For this review, use the dimensioned drawing (mm, ordinates from the lowest corner) and the shaded views. A direction names the side the tool comes from. Coordinates: 2 decimals unless noted, no trailing zeros. Write each loop counter-clockwise with the first axis right and the second up, starting at its lowest first coordinate (ties: lowest second). Pieces come first, ordered by that corner, then holes. Notation, with made-up numbers: (71.5, 28) - (97.5, 28) arc R12 ccw to (97.5, 38) - close; hole circle Ø7 at (7, 50). An arc over 180 degrees is marked (long way). One line per item, written item: value.
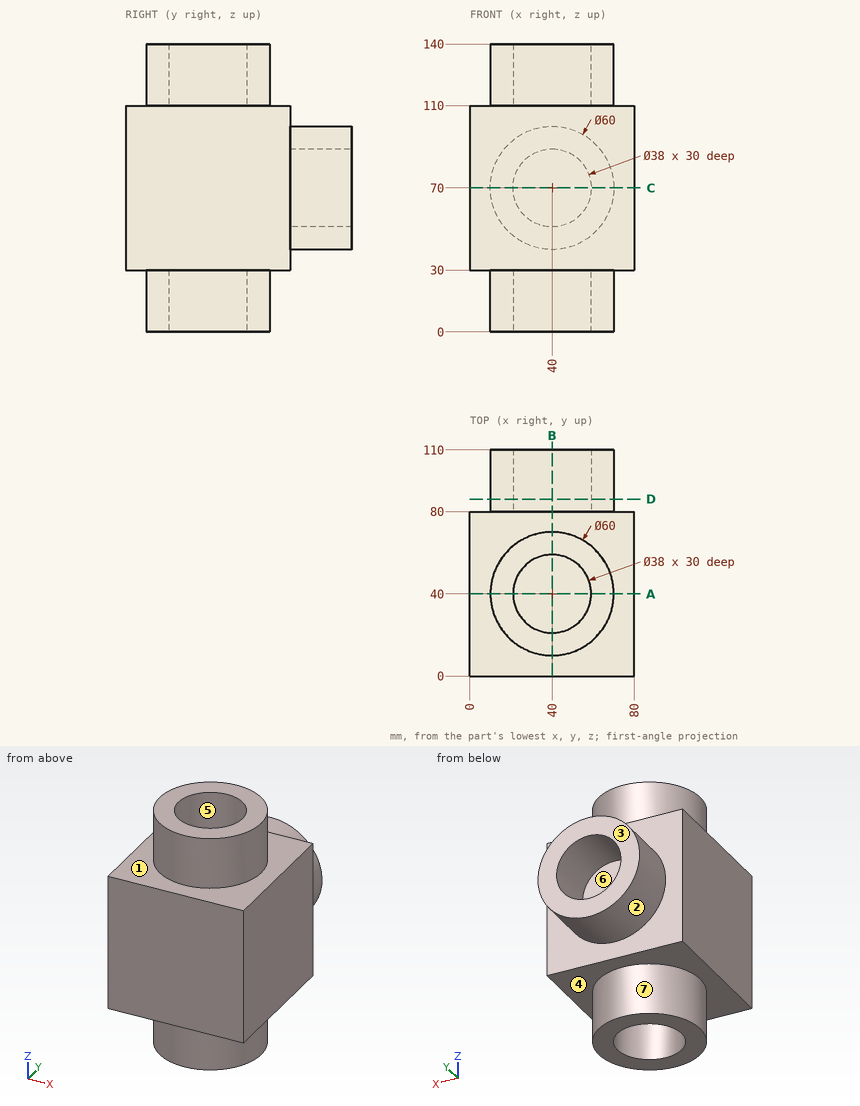
1. Consider section B-B, the plane x = 40. Write out the cut boundary in (y, z).
Answer block:
outline: (0, 30) - (10, 30) - (10, 0) - (21, 0) - (21, 30) - (59, 30) - (59, 0) - (70, 0) - (70, 30) - (80, 30) - (80, 40) - (110, 40) - (110, 51) - (80, 51) - (80, 89) - (110, 89) - (110, 100) - (80, 100) - (80, 110) - (70, 110) - (70, 140) - (59, 140) - (59, 110) - (21, 110) - (21, 140) - (10, 140) - (10, 110) - (0, 110) - close
2. Consider section D-D, the plane y = 86. Write out the cut boundary in (x, z), then the cut area to 3 significant figures.
Answer block:
outline: circle Ø60 at (40, 70); hole circle Ø38 at (40, 70)
area: 1,690 mm^2
3. For the marked faces 1, 2, 3 and 4, list the 3-axis set-ups (+Z, -Z, +X, -X, +Y, -Y) from which the entire face can be reached by the end or side of a thin tool; tool diameter is ignored.
Answer block:
face 1: +Z
face 2: +Y
face 3: +Z, -Z, +X, -X, +Y
face 4: -Z
4. Insertion check: pin 1 Ø5 at (x, z) = (43.5, 76) entering from +Y; pin 2 Ø23 at (x, y) = (40, 40) entering from -Z. Each pin has a flat end and moves straight along its axis. Give the tip position at first contact, or say it passes through.
Answer block:
pin 1: stops at y = 80
pin 2: stops at z = 30
5. Mouldability with a two-part tool opening along Y and no side actions: class the marked faces 5, 6 and 7 as released by +Y, released by -Y, zero draft, split by the parting line, or undercut.
Answer block:
face 5: undercut
face 6: released by +Y
face 7: split by the parting line
6. Wall thickness on line 1 along Y through (x, z) = (40, 15.75); line 2 along Z through (x, y) = (32.5, 31.5): over which ranges is each line inside the solid? List them lowest first.
Answer block:
line 1: y = 10 to 21, 59 to 70
line 2: z = 30 to 110
7. Consider section A-A, the plane y = 40. Write out the cut boundary in (x, z).
Answer block:
outline: (0, 30) - (10, 30) - (10, 0) - (21, 0) - (21, 30) - (59, 30) - (59, 0) - (70, 0) - (70, 30) - (80, 30) - (80, 110) - (70, 110) - (70, 140) - (59, 140) - (59, 110) - (21, 110) - (21, 140) - (10, 140) - (10, 110) - (0, 110) - close
8. Consider section C-C, the plane z = 70. Write out the cut boundary in (x, y), then the cut area to 3 significant figures.
Answer block:
outline: (0, 0) - (80, 0) - (80, 80) - (70, 80) - (70, 110) - (59, 110) - (59, 80) - (21, 80) - (21, 110) - (10, 110) - (10, 80) - (0, 80) - close
area: 7,060 mm^2
